Build history of the part. All positions in model axes, mm. A direction names the side the tool comes from. Round coordinates to 2 decimals unless told otherwise and drop trailing zeros. Order: outer loops, then holes, each group sorted by start corner. A loop starts at its lowest first (then second) coordinate and runs counter-clockwise, first axis right, second up. Notation, with made-up numbers: (-10.5, 58) -> (36.5, 58) arc R24 ccw to (36.5, 81) -> close; hole circle Ø5 at (-11, 51). An arc over 180 degrees is marked (long way). Write item = value, one per line.
from build123d import *

# Parameters (mm, degrees)
SKETCH2_W           = 130
SKETCH2_H           = 150
BOSS_EXTRUDE2_DEPTH = 35
CUT_EXTRUDE2_DEPTH  = 65
FILLET1_R           = 5


with BuildPart() as part:
    # Sketch2 → Boss-Extrude2 (new body, symmetric)
    with BuildSketch(Plane.XY):
        Rectangle(SKETCH2_W, SKETCH2_H)
    extrude(amount=BOSS_EXTRUDE2_DEPTH, both=True)

    # Sketch3 → Cut-Extrude2 (cut)
    with BuildSketch(Plane.XY.offset(35)):
        with BuildLine():
            Line((57.5, 72.5), (-57.5, 72.5))
            ThreePointArc((-57.5, 72.5), (-58.964466094, 68.964466094), (-62.5, 67.5))
            Line((-62.5, 67.5), (-62.5, -67.5))
            ThreePointArc((-62.5, -67.5), (-58.964466094, -68.964466094), (-57.5, -72.5))
            Line((-57.5, -72.5), (57.5, -72.5))
            ThreePointArc((57.5, -72.5), (58.964466094, -68.964466094), (62.5, -67.5))
            Line((62.5, -67.5), (62.5, 67.5))
            ThreePointArc((62.5, 67.5), (58.964466094, 68.964466094), (57.5, 72.5))
        make_face()
    extrude(amount=-CUT_EXTRUDE2_DEPTH, mode=Mode.SUBTRACT)

    # Fillet1
    fillet1_edges = [part.edges().sort_by_distance(p)[0] for p in [
        (65, -75, 0),
        (-65, -75, 0),
        (-65, 75, 0),
        (65, 75, 0),
    ]]
    fillet(fillet1_edges, radius=FILLET1_R)


solid = part.part
Q1. Which spindle directions (+Z, -Z, +X, -X, +Y, -Y) get a long thin tool onto all of the face, cutting with end or side? Do faces 4 (the face through (-59, -68.93, 2.95)), 5 (the face through (-64, -73, 0)). Say none if no direction does.
Check values:
face_4 = +Z
face_5 = +Z, -Z, -X, -Y
Q2. Cut at C-C, the plane y = -21.5. List the corners of the cut face in (x, z).
Check values:
outline = (-65, -35) -> (65, -35) -> (65, 35) -> (62.5, 35) -> (62.5, -30) -> (-62.5, -30) -> (-62.5, 35) -> (-65, 35) -> close
Q3. Probe probe 1 along X at (y, z) = (32, 11); probe 2 along Y at (x, z) = (-47.5, -10.5); probe 3 along Z at (x, y) = (28, -46.5). List the from-to ranges inside material, lowest first.
Check values:
probe_1 = -65 to -62.5, 62.5 to 65
probe_2 = -75 to -72.5, 72.5 to 75
probe_3 = -35 to -30
Q4. Mould opens along Y. For faces 1 (the face through (-65, -1, 0)), 2 (the face through (-64, 73, 0)), 3 (the face through (-62.5, 1, 3)) say: released by +Y, released by -Y, zero draft, split by the parting line, or undercut.
Check values:
face_1 = zero draft
face_2 = released by +Y
face_3 = undercut
Q5. Cut at B-B, the plane x = 42.5. List the corners of the cut face in (y, z).
Check values:
outline = (-75, -35) -> (75, -35) -> (75, 35) -> (72.5, 35) -> (72.5, -30) -> (-72.5, -30) -> (-72.5, 35) -> (-75, 35) -> close
Q6. Cut at A-A, the plane z = 17. List the corners of the cut face in (x, y), and give its area (3 significant figures).
Check values:
outline = (-65, -70) arc R5 ccw to (-60, -75) -> (60, -75) arc R5 ccw to (65, -70) -> (65, 70) arc R5 ccw to (60, 75) -> (-60, 75) arc R5 ccw to (-65, 70) -> close; hole (-62.5, -67.5) arc R5 cw to (-57.5, -72.5) -> (57.5, -72.5) arc R5 cw to (62.5, -67.5) -> (62.5, 67.5) arc R5 cw to (57.5, 72.5) -> (-57.5, 72.5) arc R5 cw to (-62.5, 67.5) -> close
area = 1,430 mm²
